Geometry check sheet. Reference: the model listing, model coordinates, mm. Coordinates: 2 decimals unless noted, no trailing zeros. Write each loop counter-clockwise with the first axis right and the second up, starting at its lowest first coordinate (ties: lowest second). Pieces come first, ordered by that corner, then holes.
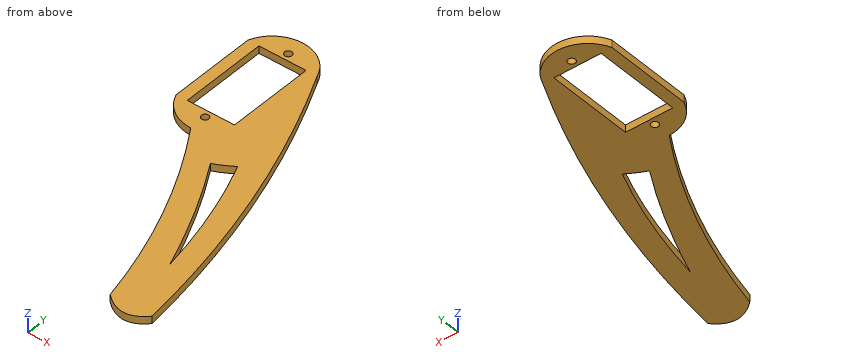
from build123d import *

# Parameters (mm, degrees)
SKETCH1_R           = 1
SKETCH1_W           = 12.8
SKETCH1_H           = 23.5
BOSS_EXTRUDE1_DEPTH = 2


with BuildPart() as part:
    # Sketch1 → Boss-Extrude1 (new body)
    with BuildSketch(Plane.XY):
        with BuildLine():
            Line((-9.4, 11.75), (-9.4, -11.75))
            ThreePointArc((-9.4, -11.75), (-5.739449267, -16.527194588), (0, -18.338255578))
            ThreePointArc((0, -18.338255578), (13.57537109, -44.028371556), (22.280776055, -71.75))
            add(Edge.make_bspline(
                [(33.607962355, -71.75), (28.503418884, -77.33913538), (22.280776055, -71.75)],
                knots=[0, 0, 0, 1, 1, 1], degree=2))
            ThreePointArc((33.607962355, -71.75), (25.161513792, -28.93962381), (9.4, 11.75))
            ThreePointArc((9.4, 11.75), (0, 18.338255578), (-9.4, 11.75))
        make_face()
        with Locations((0, -13.65)):
            Circle(SKETCH1_R, mode=Mode.SUBTRACT)
        Rectangle(SKETCH1_W, SKETCH1_H, mode=Mode.SUBTRACT)
        with Locations((0, 13.65)):
            Circle(SKETCH1_R, mode=Mode.SUBTRACT)
        with BuildLine():
            add(Edge.make_bspline(
                [(15.725665239, -21.969234099), (22.521602369, -37.712210356), (25.511369443, -56.077189315)],
                knots=[0, 0, 0, 1, 1, 1], degree=2))
            add(Edge.make_bspline(
                [(10.679903774, -24.816999203), (19.088197707, -38.847286621), (25.511369443, -56.077189315)],
                knots=[0, 0, 0, 1, 1, 1], degree=2))
            ThreePointArc((10.679903774, -24.816999203), (13.279343366, -23.528766092), (15.725665239, -21.969234099))
        make_face(mode=Mode.SUBTRACT)
    extrude(amount=BOSS_EXTRUDE1_DEPTH)


solid = part.part
1. Sectioned sample at B-B, the plane x = 5. Record the boundary of the cut face in (y, z), and give its area (3 significant figures).
Computed values:
outline: (-26.55, 0) - (-11.75, 0) - (-11.75, 2) - (-26.55, 2) - close; (11.75, 0) - (17, 0) - (17, 2) - (11.75, 2) - close
area: 40.1 mm2
2. Gauge pin test, flat ends, axial feed: pin 1 Ø1 at (y, z) = (-41.5, 0) entering from -X; pin 2 Ø1 at (x, z) = (1.5, 0.5) entering from -Y. Record the tip position at first contact, or that the pin passes through.
Computed values:
pin 1: stops at x = 12.28
pin 2: stops at y = -21.49
3. Thickness scan on line 1 along Y through (x, z) = (0, 1.2); line 2 along X through (y, z) = (-2.5, 0.3); line 3 along X through (y, z) = (-34.5, 1.75). Record the ranges inside material, lowest first.
Computed values:
line 1: y = -18.34 to -14.65, -12.65 to -11.75, 11.75 to 12.65, 14.65 to 18.34
line 2: x = -9.4 to -6.4, 6.4 to 15.86
line 3: x = 9.23 to 16.05, 20.4 to 26.7
4. Sectioned sample at C-C, the plane z = 1.25. Give the number of separate pieces and of enclosed holes in the cut face, and give its area (3 significant figures).
Computed values:
separate pieces: 1
enclosed holes: 4
area: 1,280 mm2
5. Sectioned sample at A-A, the plane y = -13.65. Record the boundary of the cut face in (x, z), and give its area (3 significant figures).
Computed values:
outline: (-8.47, 0) - (-1, 0) - (-1, 2) - (-8.47, 2) - close; (1, 0) - (20.19, 0) - (20.19, 2) - (1, 2) - close
area: 53.3 mm2
